Geometry: final body of the model. Coordinates: model frame, mm. Round coordinates to 2 decimals unless told otherwise and drop trailing zeros. Loops run counter-clockwise (first coordinate to the right, second up) from the corner with the lowest first, then second, coordinate; pieces in that order, holes last. Notation, with made-up numbers: M -28,65 L 14,65 A17 cw 14,94 Z; hole C 48,-30 d3. An arc over 180 degrees is marked long. Answer as a JSON object with one key per item and string values.
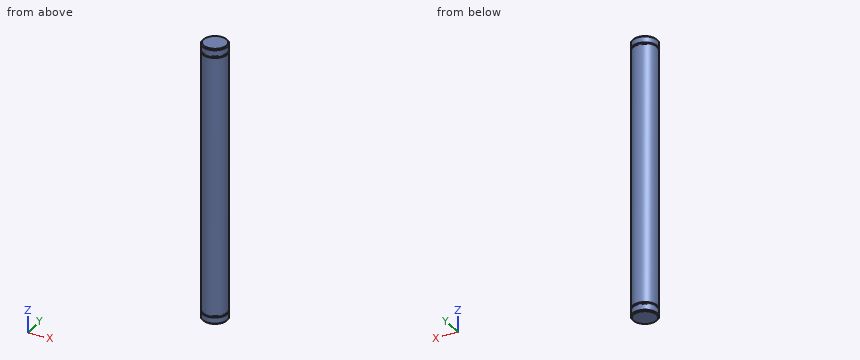
```python
from build123d import *

# Parameters (mm, degrees)
SKETCH_1_R      = 2.5
EXTRUDE_1_DEPTH = 27.75
SKETCH_2_W      = 0.35
SKETCH_2_H      = 0.2
CHAMFER_1_SIZE  = 0.2


with BuildPart() as part:
    # 草图1 → 凸台-拉伸1 (new, symmetric)
    with BuildSketch(Plane.XY):
        Circle(SKETCH_1_R)
    extrude(amount=EXTRUDE_1_DEPTH, both=True)

    # 草图2 → 切除-旋转1 (revolve, cut)
    with BuildSketch(Plane(origin=(0, 0, 0), x_dir=(0, 0, -1), z_dir=(1, 0, 0)), mode=Mode.PRIVATE) as cut_revolve_1_sk:
        with Locations((-26.175, 2.4)):
            Rectangle(SKETCH_2_W, SKETCH_2_H)
        with Locations((26.175, 2.4)):
            Rectangle(SKETCH_2_W, SKETCH_2_H)
    revolve(cut_revolve_1_sk.sketch.rotate(Axis((0, 0, 27.75), (0, 0, -1)), 90), axis=Axis((0, 0, 27.75), (0, 0, -1)), mode=Mode.SUBTRACT)

    # 倒角1
    chamfer_1_edges = [part.edges().sort_by_distance(p)[0] for p in [
        (-2.5, 0, -27.75),
        (-2.5, 0, 27.75),
    ]]
    chamfer(chamfer_1_edges, length=CHAMFER_1_SIZE)


solid = part.part
```
1) Line query: probe 1 along Z at (x, y) = (1.85, -1.6); probe 2 along X at (y, z) = (0.1, -18); probe 3 along X at (y, z) = (1, 8.5). Output: solid intervals per line, ascending.
Geometry results:
{"probe 1": "-27.6 to -26.35, -26 to 26, 26.35 to 27.6", "probe 2": "-2.5 to 2.5", "probe 3": "-2.29 to 2.29"}
2) Cut plane A-A on z = -3.5. Return the cut outline in (x, y), and give its area (3 significant figures).
Geometry results:
{"outline": "C 0,0 d5", "area": "19.6 mm2"}
3) First-contact query: pin 1 (2 mm diameter, centred on x = 2, z = 7, fed in from +Y); pin 2 (1.5 mm diameter, centred on y = 1, z = 15.5, fed in from -X); pin 3 (1 mm diameter, centred on y = -1.5, z = 10, fed in from -X). Flat tips, straight axial feed; report the tip coordinate or a pass-through.
Geometry results:
{"pin 1": "y = 2.29", "pin 2": "x = -2.49", "pin 3": "x = -2.29"}
